The listing builds one solid part. Answer for the finished solid, in the listing's coordinates (mm). Face numbers are marked on the shaded views. Give positions to 0.01 mm unless a question says otherwise; leave off trailing zeros. Write each loop counter-clockwise with the first axis right and the second up, starting at its lowest first coordinate (ties: lowest second). Pieces come first, ordered by that corner, then holes. Notation, with made-up numbers: (-2, 60) -> (54, 60) arc R20 ccw to (54, 78) -> close; hole circle Ø1 at (59.25, 36). An arc over 180 degrees is marked (long way). Put each result on its own line as item: value. Start each with the question number.
1) For a pull along X with two mould halves and no side action, classify the marked faces 1 and 2 as released by +X, released by -X, zero draft, split by the parting line, or undercut.
2) A cutting plane is placed at C-C (z = -42.5). Write down the section's boundary in (x, y), then the cut area to 3 significant figures.
3) Flat-ended cylindrical pins translate along their axes: pin 1 Ø2.5 at (y, z) = (4, -73) entering from -X; pin 2 Ø1.5 at (y, z) = (5, -62.5) entering from +X; pin 3 Ø4 at (x, y) = (-48.5, 2) entering from +Z; pin 4 Ø6 at (x, z) = (-55.5, 6) entering from -Y. Find the tip coordinate at first contact, or state that the pin passes through.
4) A cutting plane is placed at A-A (y = 6.75). Write down the section's boundary in (x, z) (3 decimals).
5) Find the intervals of material crossed by line 1 along X through (y, z) = (5.25, -4); line 2 along Z through (x, y) = (-58.5, 4.5); line 3 along X through (y, z) = (4.25, -12.5), in increasing order. Write a range as from..to.
6) A cutting plane is placed at B-B (x = 33.5). Write down the section's boundary in (y, z), then the cut area to 3 significant figures.
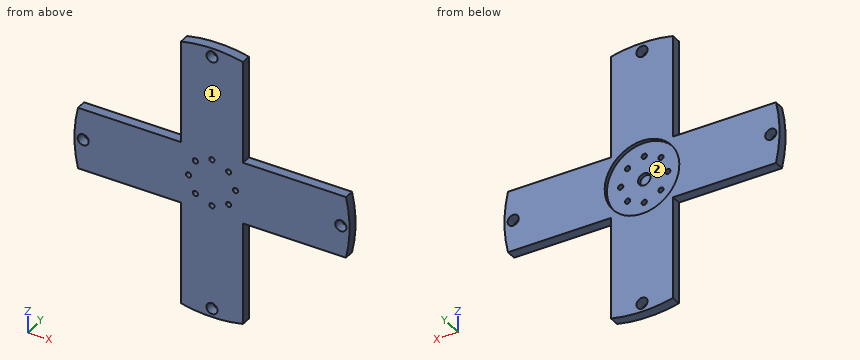
from build123d import *

# Parameters (mm, degrees)
SKETCH_1_R          = 2.1
SKETCH_1_R_2        = 4.5
EXTRUDE_1_DEPTH     = 8
SKETCH_2_R          = 30.120830341
CUT_EXTRUDE_1_DEPTH = 3
SKETCH_3_R          = 5
CUT_EXTRUDE_2_DEPTH = 3


with BuildPart() as part:
    # 草图1 → 凸台-拉伸1 (new body)
    with BuildSketch(Plane(origin=(0, 0, 0), x_dir=(1, 0, 0), z_dir=(0, 1, 0))):
        with BuildLine():
            Line((-25, 108.148046677), (-25, 25))
            Line((-25, 25), (-108.148046677, 25))
            ThreePointArc((-108.148046677, 25), (-111, 0), (-108.148046677, -25))
            Line((-108.148046677, -25), (-25, -25))
            Line((-25, -25), (-25, -108.148046677))
            ThreePointArc((-25, -108.148046677), (0, -111), (25, -108.148046677))
            Line((25, -108.148046677), (25, -25))
            Line((25, -25), (108.148046677, -25))
            ThreePointArc((108.148046677, -25), (111, 0), (108.148046677, 25))
            Line((108.148046677, 25), (25, 25))
            Line((25, 25), (25, 108.148046677))
            ThreePointArc((25, 108.148046677), (0, 111), (-25, 108.148046677))
        make_face()
        with Locations(Location((0, 19, 0), (0, 0, 270))):
            Circle(SKETCH_1_R, mode=Mode.SUBTRACT)
        with Locations(Location((13.435028843, 13.435028843, 0), (0, 0, 270))):
            Circle(SKETCH_1_R, mode=Mode.SUBTRACT)
        with Locations(Location((19, 0, 0), (0, 0, 270))):
            Circle(SKETCH_1_R, mode=Mode.SUBTRACT)
        with Locations(Location((13.435028843, -13.435028843, 0), (0, 0, 270))):
            Circle(SKETCH_1_R, mode=Mode.SUBTRACT)
        with Locations(Location((0, -19, 0), (0, 0, 270))):
            Circle(SKETCH_1_R, mode=Mode.SUBTRACT)
        with Locations(Location((-13.435028843, -13.435028843, 0), (0, 0, 270))):
            Circle(SKETCH_1_R, mode=Mode.SUBTRACT)
        with Locations(Location((-19, 0, 0), (0, 0, 270))):
            Circle(SKETCH_1_R, mode=Mode.SUBTRACT)
        with Locations(Location((-13.435028843, 13.435028843, 0), (0, 0, 270))):
            Circle(SKETCH_1_R, mode=Mode.SUBTRACT)
        with Locations(Location((0, 103.945, 0), (0, 0, 270))):
            Circle(SKETCH_1_R_2, mode=Mode.SUBTRACT)
        with Locations(Location((103.945, 0, 0), (0, 0, 270))):
            Circle(SKETCH_1_R_2, mode=Mode.SUBTRACT)
        with Locations(Location((0, -103.945, 0), (0, 0, 270))):
            Circle(SKETCH_1_R_2, mode=Mode.SUBTRACT)
        with Locations(Location((-103.945, 0, 0), (0, 0, 270))):
            Circle(SKETCH_1_R_2, mode=Mode.SUBTRACT)
    extrude(amount=EXTRUDE_1_DEPTH)

    # 草图2 → 切除-拉伸1 (cut)
    with BuildSketch(Plane(origin=(0, 8, 0), x_dir=(1, 0, 0), z_dir=(0, 1, 0))):
        with Locations(Location((0, 0, 0), (0, 0, 270))):
            Circle(SKETCH_2_R)
    extrude(amount=-CUT_EXTRUDE_1_DEPTH, mode=Mode.SUBTRACT)

    # 草图3 → 切除-拉伸2 (cut)
    with BuildSketch(Plane(origin=(0, 5, 0), x_dir=(1, 0, 0), z_dir=(0, 1, 0))):
        with Locations(Location((0, 0, 0), (0, 0, 270))):
            Circle(SKETCH_3_R)
    extrude(amount=-CUT_EXTRUDE_2_DEPTH, mode=Mode.SUBTRACT)


solid = part.part
Reply:
1. face 1: zero draft
1. face 2: undercut
2. outline: (-25, 0) -> (25, 0) -> (25, 8) -> (-25, 8) -> close
2. area: 400 mm2
3. pin 1: stops at x = -25
3. pin 2: stops at x = 25
3. pin 3: stops at z = 25
3. pin 4: stops at y = 0
4. outline: (-108.148, -25) -> (-25, -25) -> (-25, -108.148) arc R111 ccw to (25, -108.148) -> (25, -25) -> (108.148, -25) arc R111 ccw to (108.148, 25) -> (25, 25) -> (25, 108.148) arc R111 ccw to (-25, 108.148) -> (-25, 25) -> (-108.148, 25) arc R111 ccw to start; hole circle Ø9 at (-103.945, 0); hole circle Ø60.242 at (0, 0); hole circle Ø9 at (0, -103.945); hole circle Ø9 at (0, 103.945); hole circle Ø9 at (103.945, 0)
5. line 1: x = -110.93..-106.01, -101.88..-29.85, 29.85..101.88, 106.01..110.93
5. line 2: z = -25..25
5. line 3: x = -110.29..-15.32, -11.55..11.55, 15.32..110.29
6. outline: (0, -25) -> (8, -25) -> (8, 25) -> (0, 25) -> close
6. area: 400 mm2
